CAD build for the part. Positions are in the model's coordinates, mm. A direction names the side the tool comes from. Round coordinates to 2 decimals unless told otherwise and drop trailing zeros. Order: outer loops, then holes, each group sorted by start corner. A loop starts at its lowest first (then second) coordinate and runs counter-clockwise, first axis right, second up.
```python
from build123d import *

# Parameters (mm, degrees)
SKETCH_1_R      = 2.5
EXTRUDE_1_DEPTH = 150


with BuildPart() as part:
    # 草图1 → 凸台-拉伸1 (new body)
    with BuildSketch(Plane.XY):
        with BuildLine():
            ThreePointArc((-8.944458369, 9.930115847), (-9.792033903, 9.405190523), (-10.123344197, 8.464890373))
            Line((-10.123344197, 8.464890373), (-10.123344197, 3.564890373))
            Line((-10.123344197, 3.564890373), (-9.823344197, 3.564890373))
            ThreePointArc((-9.823344197, 3.564890373), (-9.681922841, 3.50631173), (-9.623344197, 3.364890373))
            Line((-9.623344197, 3.364890373), (-9.623344197, 3.064890373))
            Line((-9.623344197, 3.064890373), (-8.623344197, 3.064890373))
            ThreePointArc((-8.623344197, 3.064890373), (-8.411212162, 3.152758339), (-8.323344197, 3.364890373))
            Line((-8.323344197, 3.364890373), (-8.323344197, 5.164890373))
            ThreePointArc((-8.323344197, 5.164890373), (-8.235476231, 5.377022408), (-8.023344197, 5.464890373))
            Line((-8.023344197, 5.464890373), (-6.683344197, 5.464890373))
            Line((-6.683344197, 5.464890373), (-4.462684025, 3.244230202))
            ThreePointArc((-4.462684025, 3.244230202), (-4.137524898, 2.757595178), (-4.023344197, 2.18357003))
            Line((-4.023344197, 2.18357003), (-4.023344197, -2.253789283))
            ThreePointArc((-4.023344197, -2.253789283), (-4.137524898, -2.827814432), (-4.462684025, -3.314449455))
            Line((-4.462684025, -3.314449455), (-6.683344197, -5.535109627))
            Line((-6.683344197, -5.535109627), (-8.023344197, -5.535109627))
            ThreePointArc((-8.023344197, -5.535109627), (-8.235476231, -5.447241661), (-8.323344197, -5.235109627))
            Line((-8.323344197, -5.235109627), (-8.323344197, -3.435109627))
            ThreePointArc((-8.323344197, -3.435109627), (-8.411212162, -3.222977592), (-8.623344197, -3.135109627))
            Line((-8.623344197, -3.135109627), (-9.623344197, -3.135109627))
            Line((-9.623344197, -3.135109627), (-9.623344197, -3.435109627))
            ThreePointArc((-9.623344197, -3.435109627), (-9.681922841, -3.576530983), (-9.823344197, -3.635109627))
            Line((-9.823344197, -3.635109627), (-10.123344197, -3.635109627))
            Line((-10.123344197, -3.635109627), (-10.123344197, -8.535109627))
            ThreePointArc((-10.123344197, -8.535109627), (-9.684004369, -9.595769798), (-8.623344197, -10.035109627))
            Line((-8.623344197, -10.035109627), (-3.723344197, -10.035109627))
            Line((-3.723344197, -10.035109627), (-3.723344197, -9.735109627))
            ThreePointArc((-3.723344197, -9.735109627), (-3.664765553, -9.59368827), (-3.523344197, -9.535109627))
            Line((-3.523344197, -9.535109627), (-3.223344197, -9.535109627))
            Line((-3.223344197, -9.535109627), (-3.223344197, -8.535109627))
            ThreePointArc((-3.223344197, -8.535109627), (-3.311212162, -8.322977592), (-3.523344197, -8.235109627))
            Line((-3.523344197, -8.235109627), (-5.323344197, -8.235109627))
            ThreePointArc((-5.323344197, -8.235109627), (-5.535476231, -8.147241661), (-5.623344197, -7.935109627))
            Line((-5.623344197, -7.935109627), (-5.623344197, -6.595109627))
            Line((-5.623344197, -6.595109627), (-3.402684025, -4.374449455))
            ThreePointArc((-3.402684025, -4.374449455), (-2.916049002, -4.049290328), (-2.342023853, -3.935109627))
            Line((-2.342023853, -3.935109627), (2.09533546, -3.935109627))
            ThreePointArc((2.09533546, -3.935109627), (2.669360608, -4.049290328), (3.155995631, -4.374449455))
            Line((3.155995631, -4.374449455), (5.376655803, -6.595109627))
            Line((5.376655803, -6.595109627), (5.376655803, -7.935109627))
            ThreePointArc((5.376655803, -7.935109627), (5.288787838, -8.147241661), (5.076655803, -8.235109627))
            Line((5.076655803, -8.235109627), (3.276655803, -8.235109627))
            ThreePointArc((3.276655803, -8.235109627), (3.064523769, -8.322977592), (2.976655803, -8.535109627))
            Line((2.976655803, -8.535109627), (2.976655803, -9.535109627))
            Line((2.976655803, -9.535109627), (3.276655803, -9.535109627))
            ThreePointArc((3.276655803, -9.535109627), (3.418077159, -9.59368827), (3.476655803, -9.735109627))
            Line((3.476655803, -9.735109627), (3.476655803, -10.035109627))
            Line((3.476655803, -10.035109627), (8.376655803, -10.035109627))
            ThreePointArc((8.376655803, -10.035109627), (9.316955952, -9.703799333), (9.841881277, -8.856223799))
            ThreePointArc((9.841881277, -8.856223799), (4.018791427, 4.107025997), (-8.944458369, 9.930115847))
        make_face()
        with BuildLine():
            ThreePointArc((7.820216628, -5.531930203), (7.798494154, -5.534313715), (7.776655803, -5.535109627))
            Line((7.776655803, -5.535109627), (6.436655803, -5.535109627))
            Line((6.436655803, -5.535109627), (4.215995631, -3.314449455))
            ThreePointArc((4.215995631, -3.314449455), (3.890836504, -2.827814432), (3.776655803, -2.253789283))
            Line((3.776655803, -2.253789283), (3.776655803, 2.173084343))
            ThreePointArc((3.776655803, 2.173084343), (6.257892136, -1.4383023), (7.820216628, -5.531930203))
        make_face(mode=Mode.SUBTRACT)
        with BuildLine():
            ThreePointArc((-5.620164773, 7.908451198), (-1.52653687, 6.346126706), (2.084849773, 3.864890373))
            Line((2.084849773, 3.864890373), (-2.342023853, 3.864890373))
            ThreePointArc((-2.342023853, 3.864890373), (-2.916049002, 3.979071075), (-3.402684025, 4.304230202))
            Line((-3.402684025, 4.304230202), (-5.623344197, 6.524890373))
            Line((-5.623344197, 6.524890373), (-5.623344197, 7.864890373))
            ThreePointArc((-5.623344197, 7.864890373), (-5.622548285, 7.886728724), (-5.620164773, 7.908451198))
        make_face(mode=Mode.SUBTRACT)
        with Locations((-0.123344197, -0.035109627)):
            Circle(SKETCH_1_R, mode=Mode.SUBTRACT)
    extrude(amount=EXTRUDE_1_DEPTH)


solid = part.part
```
1. Tool access for faces 5 (the face through (-2, -2, 0)), 6 (the face through (0, -3.935, 74)), 7 (the face through (-4.023, 0, 74)): list every direction of +Z, -Z, +X, -X, +Y, -Y with a clear straight run to the whole face (end or side of a thin tool).
2. Drill centre lines: line 1 (X direction, y = -4.5, z = 127); line 2 (X direction, y = -1.25, z = 95.5); line 3 (X direction, y = 5, z = 125). Where is each one in solid material? Low to high.
3. Pin check, flat tips, straight feed: P1, Ø1.1, axis at x = 7, z = 95, coming from the +Y side; P2, Ø0.7, axis at x = -7.5, z = 69, coming from the +Y side; P3, Ø6, axis at y = -1.5, z = 82, coming from the +X side. Stop position of each tip, or through.
4. Cut at B-B, the plane z = 11.5. Give the number of separate pieces and of enclosed holes in the cut face, and give its area (3 significant figures).
5. Mould opens along Y. For faces 1 (the face through (3.777, 0, 74)), 2 (the face through (-6, -10.035, 74)), 3 (the face through (0, 3.865, 74)), 4 (the face through (-2, -2, 150)) say: released by +Y, released by -Y, zero draft, split by the parting line, or undercut.
6. Cut at A-A, the plane x = -0.5. Write the cut outline in (y, z), and give its area (3 significant figures).
Outcome:
1. face 5: -Z, +X, -X, +Y, -Y
1. face 6: +Z, -Z, -Y
1. face 7: +Z, -Z, -X
2. line 1: x = -10.12 to -8.32, -5.65 to -3.53, 3.28 to 5.4, 7.53 to 9.1
2. line 2: x = -4.02 to -2.31, 2.06 to 3.78, 6.16 to 7.84
2. line 3: x = -10.12 to -8.32, -6.22 to -4.1, 0.66 to 3.07
3. P1: stops at y = 1.16
3. P2: stops at y = 9.84
3. P3: stops at x = 9.1
4. separate pieces: 1
4. enclosed holes: 3
4. area: 160 mm2
5. face 1: undercut
5. face 2: released by -Y
5. face 3: undercut
5. face 4: zero draft
6. outline: (-3.94, 0) - (-2.51, 0) - (-2.51, 150) - (-3.94, 150) - close; (2.44, 0) - (3.86, 0) - (3.86, 150) - (2.44, 150) - close; (5.76, 0) - (7.5, 0) - (7.5, 150) - (5.76, 150) - close
6. area: 688 mm2
